Read the model definition and answer for the solid it produces. Units are mm, in the model's axes. A direction names the side the tool comes from. Coordinates: 2 decimals unless noted, no trailing zeros. Write each loop counter-clockwise with the first axis right and the second up, starting at its lowest first coordinate (ties: lowest second). Pieces come first, ordered by that corner, then holes. Notation, with made-up numbers: (-19.5, -14) - (0.5, -14) arc R26 ccw to (0.5, 21) - close; hole circle Ø10 at (77, 55.25). An arc over 180 degrees is marked (long way). Return JSON: item names as keys, results as strings.
```python
from build123d import *

# Parameters (mm, degrees)
SKETCH_1_W          = 100
SKETCH_1_H          = 100
EXTRUDE_1_DEPTH     = 6
SKETCH_2_W          = 7
SKETCH_2_H          = 6
EXTRUDE_2_DEPTH     = 6
CUT_EXTRUDE_1_DEPTH = 7


with BuildPart() as part:
    # Эскиз1 → Бобышка-Вытянуть1 (new body)
    with BuildSketch(Plane.XY):
        Rectangle(SKETCH_1_W, SKETCH_1_H)
    extrude(amount=EXTRUDE_1_DEPTH)

    # Эскиз2 → Бобышка-Вытянуть2 (add)
    with BuildSketch(Plane.XY.offset(6)):
        with Locations((-9.531849908, 53)):
            Rectangle(SKETCH_2_W, SKETCH_2_H)
        with Locations((9.531849908, 53)):
            Rectangle(SKETCH_2_W, SKETCH_2_H)
    extrude(amount=-EXTRUDE_2_DEPTH)

    # Эскиз3 → Вырез-Вытянуть1 (cut, through all)
    with BuildSketch(Plane.XY.offset(6)):
        Polygon((-2.1, 45), (-3.6, 45), (-3.6, 42.6), (-2.1, 42.6), (-2.1, 37.5), (2.1, 37.5), (2.1, 42.6), (3.6, 42.6), (3.6, 45), (2.1, 45), (2.1, 50), (-2.1, 50), align=None)
    extrude(amount=-CUT_EXTRUDE_1_DEPTH, mode=Mode.SUBTRACT)


solid = part.part
```
(1) Determine the mould class of faces 6 (the face through (-13.032, 53, 3)), 7 (the face through (-3.6, 44, 3)), 8 (the face through (-4, 50, 3)), 9 (the face through (3.6, 44, 3)) for opening direction Y: +Y half, -Y half, draft (parallel to the pull), parting line (faces both ways), or undercut.
Answer:
{"face 6": "draft", "face 7": "undercut", "face 8": "+Y half", "face 9": "undercut"}
(2) Which of the six approach directions +Z, -Z, +X, -X, +Y, -Y give full straight-line access (tool end or side, diameter ignored) to faces 1 (the face through (0, 37.5, 3)), 2 (the face through (-32, 50, 3)), 3 (the face through (-1, 4, 0)), 4 (the face through (31, 50, 3)), 5 (the face through (-1, -50, 3))?
Answer:
{"face 1": "+Z, -Z, +Y", "face 2": "+Z, -Z, -X, +Y", "face 3": "-Z, +X, -X, +Y, -Y", "face 4": "+Z, -Z, +X, +Y", "face 5": "+Z, -Z, +X, -X, -Y"}
(3) Flat-ended cylindrical pins translate along their axes: P1, Ø2, axis at x = -4, z = 3.5, coming from the +Y side; P2, Ø1, axis at x = 29.5, y = -24, coming from the -Z side. Find the tip coordinate at first contact, or state that the pin passes through.
Answer:
{"P1": "y = 50", "P2": "z = 0"}
(4) A cutting plane is placed at C-C (x = -19.5). Determine the outline of the cut face in (y, z), and give its area (3 significant figures).
Answer:
{"outline": "(-50, 0) - (50, 0) - (50, 6) - (-50, 6) - close", "area": "600 mm²"}
(5) A cutting plane is placed at B-B (z = 0.9). Determine the outline of the cut face in (x, y), and give its area (3 significant figures).
Answer:
{"outline": "(-50, -50) - (50, -50) - (50, 50) - (13.03, 50) - (13.03, 56) - (6.03, 56) - (6.03, 50) - (2.1, 50) - (2.1, 45) - (3.6, 45) - (3.6, 42.6) - (2.1, 42.6) - (2.1, 37.5) - (-2.1, 37.5) - (-2.1, 42.6) - (-3.6, 42.6) - (-3.6, 45) - (-2.1, 45) - (-2.1, 50) - (-6.03, 50) - (-6.03, 56) - (-13.03, 56) - (-13.03, 50) - (-50, 50) - close", "area": "10,000 mm²"}
(6) Straight lines are drawn through the part: line 1 (Y direction, x = -18.5, z = 3.35); line 2 (X direction, y = 51.5, z = 2). For each, find the intervals that lie inside material, in ascending order. Write a range as from..to.
Answer:
{"line 1": "-50..50", "line 2": "-13.03..-6.03, 6.03..13.03"}
(7) A cutting plane is placed at A-A (y = 41). Determine the outline of the cut face in (x, z).
Answer:
{"outline": "(-50, 0) - (-2.1, 0) - (-2.1, 6) - (-50, 6) - close; (2.1, 0) - (50, 0) - (50, 6) - (2.1, 6) - close"}
